Geometry: see drawing. Coordinates: mm, zero at the bounding-box minimum. A direction names the side the tool comes from. Give positions to 0.01 mm unless a question says otherwise; leave off trailing zeros. Order: outer loops, then holes, each group sorted by start corner. A loop starts at its lowest first (then second) coordinate and runs counter-clockwise, first axis right, second up. Notation, with made-up numbers: M 9.5,22 L 33.5,22 A30 ccw 33.5,46 Z; hole C 19.25,80 d7. An arc over 180 degrees is marked long. Return JSON: item names as keys, results as strings.
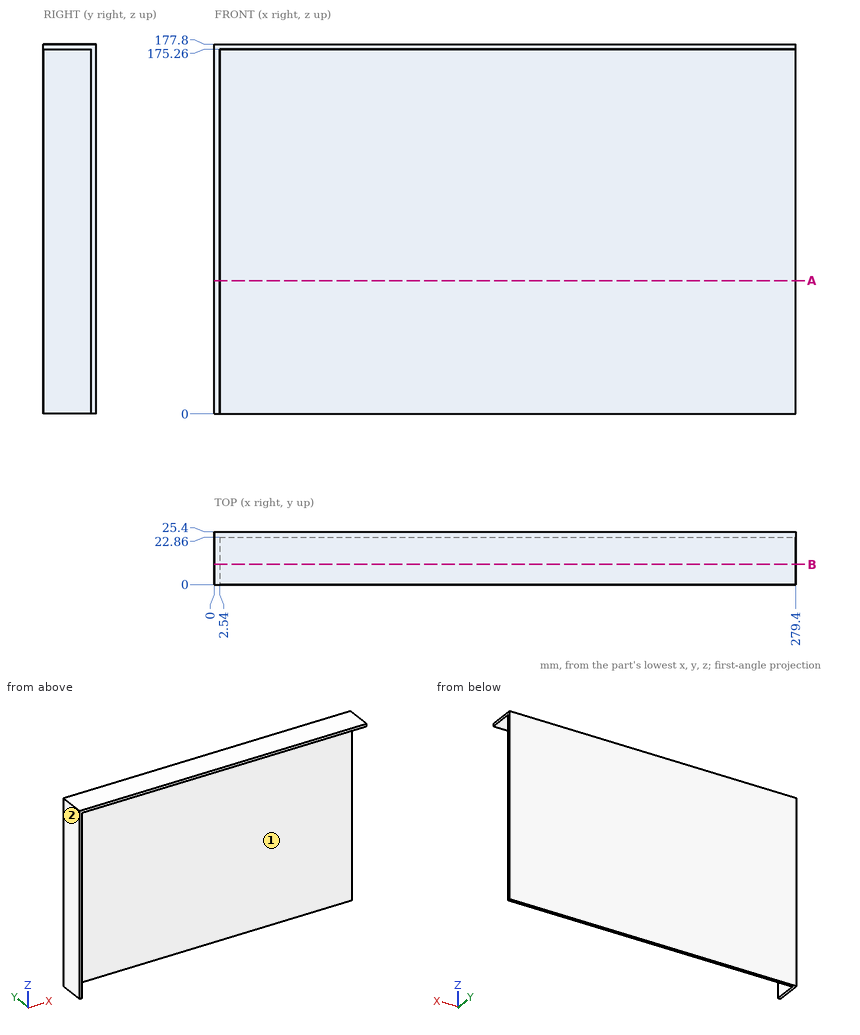
1. Set-up query: the marked faces 1 and 2. Return all of +Z, -Z, +X, -X, +Y, -Y with unobstructed straight access to the full face (end or side cutting, diameter ignored); none if empty.
Evaluation:
{"face 1": "-Z, +X, -Y", "face 2": "+Z, -Z, -X, +Y, -Y"}
2. Section query A-A (z = 64). Return loops of the section in (x, y), then the cut area to 3 significant figures.
Evaluation:
{"outline": "M 0,0 L 2.54,0 L 2.54,22.86 L 279.4,22.86 L 279.4,25.4 L 0,25.4 Z", "area": "768 mm^2"}
3. Section query B-B (y = 9.75). Return loops of the section in (x, z), then the cut area to 3 significant figures.
Evaluation:
{"outline": "M 0,0 L 2.54,0 L 2.54,175.26 L 279.4,175.26 L 279.4,177.8 L 0,177.8 Z", "area": "1,150 mm^2"}
4. Ray query, probe 1 along Z at (x, y) = (247.5, 13.25); probe 2 along X at (y, z) = (7, 162.5); probe 3 along Y at (x, z) = (259, 147). Return the intervals inside material, ascending.
Evaluation:
{"probe 1": "z = 175.26 to 177.8", "probe 2": "x = 0 to 2.54", "probe 3": "y = 22.86 to 25.4"}
5. First-contact query: pin 1 (11.5 mm diameter, centred on x = 139.5, y = 6.5, fed in from -Z); pin 2 (8 mm diameter, centred on x = 203, z = 134.5, fed in from -Y); pin 3 (8 mm diameter, centred on y = 11.5, z = 107.5, fed in from -X). Flat tips, straight axial feed; report the tip coordinate or a pass-through.
Evaluation:
{"pin 1": "stops at z = 175.26", "pin 2": "stops at y = 22.86", "pin 3": "stops at x = 0"}
